```python
from build123d import *

# Parameters (mm, degrees)
BOSS_EXTRUDE1_DEPTH           = 3.175
CONVERT_SOLID1_START          = 2.588
CONVERT_SOLID1_DEPTH          = 0.587
EDGE_FLANGE1_STRIP_W          = 18.352
EDGE_FLANGE1_STRIP_H          = 2.588
EDGE_FLANGE1_STRIP_CUT_DEPTH  = 16.036353891
EDGE_FLANGE1_RELIEF_W         = 19.646
EDGE_FLANGE1_RELIEF_H         = 1.294
EDGE_FLANGE1_RELIEF_CUT_DEPTH = 2.588
EDGE_FLANGE1_DEPTH            = 16.036353891
SKETCH9_R                     = 3.5
CUT_EXTRUDE1_DEPTH            = 47.081558227
CUT_EXTRUDE2_DEPTH            = 41.148221328
M4_CLEARANCE_HOLE1_D          = 4.5
BOSS_EXTRUDE2_DEPTH           = 2.588
SKETCH19_R                    = 7.25
CUT_EXTRUDE3_DEPTH            = 41.148221328
SKETCH20_W                    = 2
SKETCH20_H                    = 21.253234492
CUT_EXTRUDE4_DEPTH            = 10


# Read off the part's stored shape, not the designer's step: Convert-Solid1
# Sheet-metal steps are written as plain solids
with BuildPart() as part:
    # Sketch1 → Boss-Extrude1 (new body)
    with BuildSketch(Plane(origin=(0, 0, 0), x_dir=(1, 0, 0), z_dir=(0, 1, 0))):
        with BuildLine():
            Line((0, 14.5), (-27, 14.5))
            Line((-27, 14.5), (-27, -4.086))
            Line((-27, -4.086), (-19.43303559, -4.086))
            Line((-19.43303559, -4.086), (-19.43303559, -14.223687844))
            Line((-19.43303559, -14.223687844), (-7.832786234, -25.296124838))
            Line((-7.832786234, -25.296124838), (0, -25.296124838))
            Line((0, -25.296124838), (0, -14.5))
            ThreePointArc((0, -14.5), (14.5, 0), (0, 14.5))
        make_face()
    extrude(amount=BOSS_EXTRUDE1_DEPTH)

    # Convert-Solid1 outline → Convert-Solid1 (cut)
    with BuildSketch(Plane(origin=(0, 0, 0), x_dir=(1, 0, 0), z_dir=(0, 1, 0)).offset(CONVERT_SOLID1_START)):
        with BuildLine():
            Line((0, 14.5), (-27, 14.5))
            Line((-27, 14.5), (-27, -4.086))
            Line((-27, -4.086), (-19.43303559, -4.086))
            Line((-19.43303559, -4.086), (-19.43303559, -14.223687844))
            Line((-19.43303559, -14.223687844), (-7.832786234, -25.296124838))
            Line((-7.832786234, -25.296124838), (0, -25.296124838))
            Line((0, -25.296124838), (0, -14.5))
            ThreePointArc((0, -14.5), (14.5, 0), (0, 14.5))
        make_face()
    extrude(amount=CONVERT_SOLID1_DEPTH, mode=Mode.SUBTRACT)

    # Edge-Flange1 strip (across the edge) → Edge-Flange1 strip cut (cut)
    with BuildSketch(Plane(origin=(-7.832786234, 0, 25.296124838), x_dir=(0.6904585088002791, -3.4914813388431334e-15, -0.7233719980931629), z_dir=(-0.7233719980931629, 0, -0.6904585088002791))):
        with Locations((-2.588, -1.294)):
            Rectangle(EDGE_FLANGE1_STRIP_W, EDGE_FLANGE1_STRIP_H)
    extrude(amount=EDGE_FLANGE1_STRIP_CUT_DEPTH, mode=Mode.SUBTRACT)

    # Edge-Flange1 relief (on the sheet) → Edge-Flange1 relief cut (cut)
    with BuildSketch(Plane(origin=(-3.284045578, 0, 20.530550115), x_dir=(0.6904585088002791, -6.982962677686267e-15, -0.7233719980931629), z_dir=(0, -1, 0))):
        with Locations((-8.529, 0.647)):
            Rectangle(EDGE_FLANGE1_RELIEF_W, EDGE_FLANGE1_RELIEF_H)
        with Locations((-8.529, -16.683353891)):
            Rectangle(EDGE_FLANGE1_RELIEF_W, EDGE_FLANGE1_RELIEF_H)
    extrude(amount=-EDGE_FLANGE1_RELIEF_CUT_DEPTH, mode=Mode.SUBTRACT)

    # Edge-Flange1 section (across the edge) → Edge-Flange1 (add)
    with BuildSketch(Plane(origin=(-7.832786234, 0, 25.296124838), x_dir=(0.6904585088002791, -3.4914813388431334e-15, -0.7233719980931629), z_dir=(-0.7233719980931629, 0, -0.6904585088002791))):
        with BuildLine():
            Line((0, 4), (0, 13))
            Line((0, 13), (2.588, 13))
            Line((2.588, 13), (2.588, 4))
            ThreePointArc((2.588, 4), (3.759572875, 1.171572875), (6.588, 0))
            Line((6.588, 0), (6.588, -2.588))
            ThreePointArc((6.588, -2.588), (1.929580526, -0.658419474), (0, 4))
        make_face()
    extrude(amount=EDGE_FLANGE1_DEPTH)

    # Sketch9 → Cut-Extrude1 (cut, through all)
    with BuildSketch(Plane(origin=(-16.368508108, 0, 17.148779057), x_dir=(0.7233719980931632, 3.1973878914611357e-15, 0.6904585088002789), z_dir=(-0.6904585088002789, 3.4046985453530564e-15, 0.7233719980931632))):
        with Locations(Location((3.78172946, -7.5, 0), (0, 0, 90))):
            Circle(SKETCH9_R)
    extrude(amount=-CUT_EXTRUDE1_DEPTH, mode=Mode.SUBTRACT)

    # Sketch10 → Cut-Extrude2 (cut, through all)
    with BuildSketch(Plane(origin=(0, 2.588, 0), x_dir=(1, 0, 0), z_dir=(0, 1, 0))):
        Polygon((-19.43303559, -4.086), (-17.470094505, -4.086), (-14.926884989, -7.628616445), (-19.43303559, -12.349570886), align=None)
        Polygon((0, -25.296124838), (-7.832786234, -25.296124838), (0, -17.08995726), align=None)
    extrude(amount=-CUT_EXTRUDE2_DEPTH, mode=Mode.SUBTRACT)

    # M4 Clearance Hole1 (through all)
    with Locations(Plane(origin=(0, 2.588, 0), x_dir=(1, 0, 0), z_dir=(0, 1, 0))):
        with Locations((-22, 7.707), (-14, 2.707)):
            Hole(M4_CLEARANCE_HOLE1_D / 2)

    # Sketch17 → Boss-Extrude2 (add)
    with BuildSketch(Plane(origin=(0, 2.588, 0), x_dir=(1, 0, 0), z_dir=(0, 1, 0))):
        Polygon((-1.098945785, -18.241288728), (4.611253989, -11.842333594), (-0.672962036, -12.348247452), align=None)
    extrude(amount=-BOSS_EXTRUDE2_DEPTH)

    # Sketch19 → Cut-Extrude3 (cut, through all)
    with BuildSketch(Plane(origin=(0, 2.588, 0), x_dir=(1, 0, 0), z_dir=(0, 1, 0))):
        with Locations(Location((0, 0, 0), (0, 0, 270))):
            Circle(SKETCH19_R)
    extrude(amount=-CUT_EXTRUDE3_DEPTH, mode=Mode.SUBTRACT)

    # Sketch20 → Cut-Extrude4 (cut)
    with BuildSketch(Plane(origin=(0, 2.588, 0), x_dir=(1, 0, 0), z_dir=(0, 1, 0))):
        with Locations((-27, 5.207)):
            Rectangle(SKETCH20_W, SKETCH20_H)
    extrude(amount=-CUT_EXTRUDE4_DEPTH, mode=Mode.SUBTRACT)


solid = part.part
```
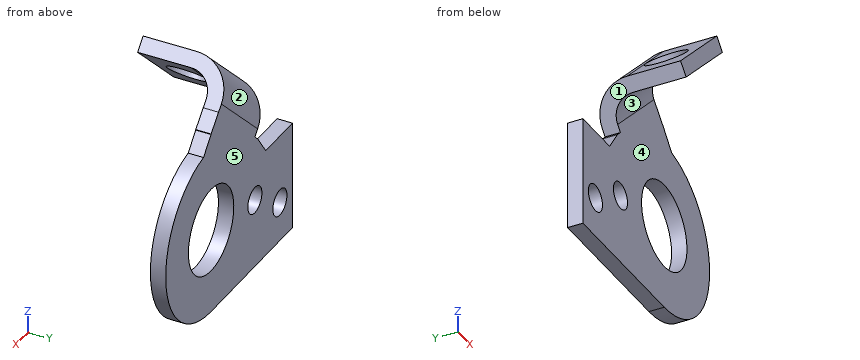
Check sheet for the modelled part. Datum: model origin and axes. Units: mm. Face numbers are marked on the shaded views. A direction names the side the tool comes from. Give positions to 0.01 mm unless a question says otherwise; leave off trailing zeros. Order: outer loops, then holes, each group sorted by start corner. A loop starts at its lowest first (then second) coordinate and runs counter-clockwise, first axis right, second up. Notation, with made-up numbers: (3, 31) -> (62, 31) arc R19 ccw to (62, 55) -> close; hole circle Ø6 at (63, -30). An arc over 180 degrees is marked (long way). Use CSV: the item, a comma, the result in double quotes. Start each with the question number.
1) Sectioned sample at C-C, the plane z = -1.5. Record the boundary of the cut face in (x, y), plus the area to 3 significant figures.
2) Sectioned sample at B-B, the plane y = -8.5. Record the boundary of the cut face in (x, z).
3) Sectioned sample at A-A, the plane x = -22. Record the boundary of the cut face in (y, z).
4) Go/stop test with flat-tipped pins: P1, Ø16.5, axis at x = 0, z = 0, coming from the -Y side; P2, Ø0.8, axis at x = -22.5, y = 2, coming from the +Z side; P3, Ø1.5, axis at y = 0, z = 9.5, coming from the +X side; P4, Ø4, axis at x = -14, z = -2.707, coming from the +Y side (3 decimals). Record where each tip stops, or that it passes through.
5) Sectioned sample at D-D, the plane y = 1.5. Record the boundary of the cut face in (x, z), plus the area to 3 significant figures.
6) Mould release check, pull along Z, two halves, no side actions. Record for the marked faces 1, 2 and 3: released by +Z, released by -Z, zero draft, split by the parting line, or undercut.
7) Set-up check for the marked faces 4 and 5: record each of +Z, -Z, +X, -X, +Y, -Y from which the full face is reachable in a straight line by a thin tool's end or side.
8) Material ranges on line 1 (Z direction, x = -22, y = 1.65); line 2 (X direction, y = 1.25, z = -2); line 3 (Y direction, x = -11.5, z = 19.5), recorded low to high. Write a range as from..to.
Recorded:
1,outline,"(-26, 0) -> (-15.9, 0) -> (-15.9, 2.59) -> (-26, 2.59) -> close; (-12.1, 0) -> (-7.09, 0) -> (-7.09, 2.59) -> (-12.1, 2.59) -> close; (7.09, 0) -> (14.42, 0) -> (14.42, 2.59) -> (7.09, 2.59) -> close"
1,area,"58.1 mm2"
2,outline,"(-19.43, 14.22) -> (-17.65, 12.35) -> (-14.27, 15.57) -> (-16.06, 17.44) -> close; (-11.21, 22.08) -> (-9.42, 20.2) -> (-6.05, 23.42) -> (-7.83, 25.3) -> close"
3,outline,"(0, -14.5) -> (2.59, -14.5) -> (2.59, -9.96) -> (0, -9.96) -> close; (0, -5.46) -> (2.59, -5.46) -> (2.59, 4.09) -> (0, 4.09) -> close"
4,P1,"y = 0"
4,P2,"z = 4.09"
4,P3,"x = 11.56"
4,P4,"through"
5,outline,"(-26, -14.5) -> (0, -14.5) arc R14.5 ccw to (2.42, 14.3) -> (0, 17.01) -> (0, 17.09) -> (-5.79, 23.15) -> (-17.39, 12.08) -> (-13.99, 8.52) -> (-14.93, 7.63) -> (-17.47, 4.09) -> (-26, 4.09) -> close; hole circle Ø4.5 at (-22, -7.71); hole circle Ø4.5 at (-14, -2.71); hole circle Ø14.5 at (0, 0)"
5,area,"856 mm2"
6,face 1,"undercut"
6,face 2,"released by +Z"
6,face 3,"released by -Z"
7,face 4,"-Z, +X, -Y"
7,face 5,"+Z, -Z, +X, -X, +Y"
8,line 1,"-14.5..-9.96, -5.46..4.09"
8,line 2,"-26..-16.14, -11.86..-6.97, 6.97..14.36"
8,line 3,"-13..-10.72, -4.28..0.37"
